Work out the finished part from the listing and answer in its coordinate system (mm). A direction names the side the tool comes from. Give positions to 0.01 mm unless a question says otherwise; leave off trailing zeros. Loops run counter-clockwise (first coordinate to the right, second up) from the corner with the lowest first, then second, coordinate; pieces in that order, holes last.
```python
from build123d import *

# Parameters (mm, degrees)
F1_DEPTH = 60
F3_DEPTH = 60.001
F5_DEPTH = 100.001


with BuildPart() as f1:
    # F0 (on Top) → F1 (new body)
    with BuildSketch(Plane.XY):
        Polygon((0, 60), (0, 0), (20, 0), (20, 15), (55, 15), (55, 0), (70, 0), (70, 20), (100, 20), (100, 60), align=None)
    extrude(amount=F1_DEPTH)

    # F2 (on face) → F3 (cut, through all)
    with BuildSketch(Plane.XZ):
        Polygon((0, 60), (0, 40), (15.3589838486, 40), (20, 42.6794919243), (20, 60), align=None)
        Polygon((20, 60), (20, 42.6794919243), (50, 60), align=None)
        Polygon((100, 60), (75, 60), (100, 35), align=None)
    extrude(amount=-F3_DEPTH, mode=Mode.SUBTRACT)

    # F4 (on face) → F5 (cut, through all)
    with BuildSketch(Plane.YZ.offset(100)):
        Polygon((27.2727272727, 35), (50, 60), (0, 60), (0, 5), (20, 27), (20, 35), align=None)
        Polygon((20, 27), (27.2727272727, 35), (20, 35), align=None)
    extrude(amount=-F5_DEPTH, mode=Mode.SUBTRACT)


solid = f1.part
```
Q1. Section B-B on z = 8.5 is taken. Give the vertices of the cut face in (x, y), plus the area to 3 significant figures.
Q2. Section A-A on y = 4 is taken. Give the vertices of the cut face in (x, z), plus the area to 3 significant figures.
Q3. Section D-D on y = 10.5 is taken. Give the vertices of the cut face in (x, z), plus the area to 3 significant figures.
Q4. Determine the mould class of faces 1 (the face through (20, 9, 8)), 2 (the face through (90, 47, 45)), 3 (the face through (55, 9, 8)), 4 (the face through (0, 37, 15)) for opening direction X: +X half, -X half, draft (parallel to the pull), parting line (faces both ways), or undercut.
Q5. Given pin 1 (1.5 mm diameter, centred on x = 78, y = 38.5, fed in from +Z) (3 decimals); pin 2 (4 mm diameter, centred on x = 65, y = 10.5, fed in from +Z); pin 3 (4 mm diameter, centred on x = 75, z = 47.5, fed in from -Y), each flat-ended and moving along its own axis, determine where each tip first touches the part or whether it passes through.
Q6. Section C-C on x = 10 is taken. Give the vertices of the cut face in (y, z).
Q7. Consider line 1 along Y through (x, z) = (87.5, 35); line 2 along Y through (x, z) = (34.5, 4); line 3 along Z through (x, y) = (14, 50.5). Determine where each line is inside the solid, lowest interval first.
Q8. Which of the six approach directions +Z, -Z, +X, -X, +Y, -Y give full straight-line access (tool end or side, diameter ignored) to faces 5 (the face through (37, 15, 11)), 6 (the face through (62, 55, 60)), 7 (the face through (85, 20, 13)), 8 (the face through (8, 46, 40))?
Check result:
1. outline: (0, 3.18) - (20, 3.18) - (20, 15) - (55, 15) - (55, 3.18) - (70, 3.18) - (70, 20) - (100, 20) - (100, 60) - (0, 60) - close
1. area: 4,760 mm2
2. outline: (0, 0) - (20, 0) - (20, 9.4) - (0, 9.4) - close; (55, 0) - (70, 0) - (70, 9.4) - (55, 9.4) - close
2. area: 329 mm2
3. outline: (0, 0) - (20, 0) - (20, 16.55) - (0, 16.55) - close; (55, 0) - (70, 0) - (70, 16.55) - (55, 16.55) - close
3. area: 579 mm2
4. face 1: undercut
4. face 2: +X half
4. face 3: undercut
4. face 4: -X half
5. pin 1: stops at z = 48.175
5. pin 2: stops at z = 18.75
5. pin 3: stops at y = 36.82
6. outline: (0, 0) - (60, 0) - (60, 40) - (31.82, 40) - (0, 5) - close
7. line 1: y = 27.27 to 60
7. line 2: y = 15 to 60
7. line 3: z = 0 to 40
8. face 5: +Z, -Z, -Y
8. face 6: +Z, +X, -X, +Y, -Y
8. face 7: +Z, -Z, +X, -Y
8. face 8: +Z, -X, +Y, -Y
